Could you check a few things on this model? Use its own coordinates, in mm. A direction names the side the tool comes from. Give positions to 0.01 mm unless a question says otherwise; leave off trailing zeros. Loops run counter-clockwise (first coordinate to the right, second up) from the corner with the lowest first, then second, coordinate; pieces in that order, holes last. Notation, with made-up numbers: (82.5, 62) - (140.5, 62) arc R14 ccw to (140.5, 68) - close; hole circle Ø6 at (41.5, 86). An arc over 180 degrees is marked (long way). Use CSV: the item, a comma, the result in double quotes.
from build123d import *

# Parameters (mm, degrees)
EXTRUDE_1_DEPTH     = 20
SKETCH_2_R          = 1.5
CUT_EXTRUDE_1_DEPTH = 4
SKETCH_3_R          = 4
CUT_EXTRUDE_2_DEPTH = 4
SKETCH_4_R          = 1.5
CUT_EXTRUDE_3_DEPTH = 20
SKETCH_5_W          = 3
SKETCH_5_H          = 20
CUT_EXTRUDE_4_DEPTH = 8
SKETCH_6_W          = 20
SKETCH_6_H          = 27
CUT_EXTRUDE_5_DEPTH = 1
SKETCH_7_W          = 18
SKETCH_7_H          = 20
CUT_EXTRUDE_6_DEPTH = 1


with BuildPart() as part:
    # 草图1 → 凸台-拉伸1 (new body)
    with BuildSketch(Plane.XY):
        Polygon((0, 0), (0, 38), (3, 38), (3, 3), (20, 3), (20, 0), align=None)
    extrude(amount=EXTRUDE_1_DEPTH)

    # 草图2 → 切除-拉伸1 (cut, through all)
    with BuildSketch(Plane(origin=(0, 3, 0), x_dir=(1, 0, 0), z_dir=(0, 1, 0))):
        with Locations((16, -16)):
            Circle(SKETCH_2_R)
        with Locations((16, -4)):
            Circle(SKETCH_2_R)
    extrude(amount=-CUT_EXTRUDE_1_DEPTH, mode=Mode.SUBTRACT)

    # 草图3 → 切除-拉伸2 (cut, through all)
    with BuildSketch(Plane(origin=(3, 0, 0), x_dir=(0, 0, -1), z_dir=(1, 0, 0))):
        with Locations((-10, 18)):
            Circle(SKETCH_3_R)
    extrude(amount=-CUT_EXTRUDE_2_DEPTH, mode=Mode.SUBTRACT)

    # 草图4 → 切除-拉伸3 (cut)
    with BuildSketch(Plane(origin=(0, 3, 0), x_dir=(1, 0, 0), z_dir=(0, 1, 0))):
        with Locations((8, -16)):
            Circle(SKETCH_4_R)
        with Locations((8, -4)):
            Circle(SKETCH_4_R)
    extrude(amount=-CUT_EXTRUDE_3_DEPTH, mode=Mode.SUBTRACT)

    # 草图5 → 切除-拉伸4 (cut)
    with BuildSketch(Plane(origin=(0, 38, 0), x_dir=(1, 0, 0), z_dir=(0, 1, 0))):
        with Locations((1.5, -10)):
            Rectangle(SKETCH_5_W, SKETCH_5_H)
    extrude(amount=-CUT_EXTRUDE_4_DEPTH, mode=Mode.SUBTRACT)

    # 草图6 → 切除-拉伸5 (cut)
    with BuildSketch(Plane(origin=(3, 0, 0), x_dir=(0, 0, -1), z_dir=(1, 0, 0))):
        with Locations((-10, 16.5)):
            Rectangle(SKETCH_6_W, SKETCH_6_H)
    extrude(amount=-CUT_EXTRUDE_5_DEPTH, mode=Mode.SUBTRACT)

    # 草图7 → 切除-拉伸6 (cut)
    with BuildSketch(Plane(origin=(0, 3, 0), x_dir=(1, 0, 0), z_dir=(0, 1, 0))):
        with Locations((11, -10)):
            Rectangle(SKETCH_7_W, SKETCH_7_H)
    extrude(amount=-CUT_EXTRUDE_6_DEPTH, mode=Mode.SUBTRACT)


solid = part.part
1) Suppose I cut it at D-D (z = 10). Please give me the cut outline in (x, y).
Answer below:
outline,"(0, 0) - (20, 0) - (20, 2) - (2, 2) - (2, 14) - (0, 14) - close; (0, 22) - (2, 22) - (2, 30) - (0, 30) - close"
2) Suppose I cut it at C-C (x = 16). Please give me the cut outline in (y, z).
Answer below:
outline,"(0, 0) - (2, 0) - (2, 2.5) - (0, 2.5) - close; (0, 5.5) - (2, 5.5) - (2, 14.5) - (0, 14.5) - close; (0, 17.5) - (2, 17.5) - (2, 20) - (0, 20) - close"
3) Suppose I cut it at A-A (z = 16). Please give me the cut outline in (x, y).
Answer below:
outline,"(0, 0) - (6.5, 0) - (6.5, 2) - (2, 2) - (2, 30) - (0, 30) - close; (9.5, 0) - (14.5, 0) - (14.5, 2) - (9.5, 2) - close; (17.5, 0) - (20, 0) - (20, 2) - (17.5, 2) - close"
4) We'd pull the mould along Z, two halves only. Please class faces 1 (the cylindrical face through (14.5, 1.01, 15.93)), 2 (the flat face through (2, 13, 10)), 3 (the flat face through (1, 10, 0)): +Z half, -Z half, draft (parallel to the pull), parting line (faces both ways), or undercut.
Answer below:
face 1,"undercut"
face 2,"draft"
face 3,"-Z half"
5) Which directions (+Z, -Z, +X, -X, +Y, -Y) give clear straight access to the entire face, cutting with the end or side of a thin tool? Please do faces 4 (the flat face through (11, 2, 10)), 5 (the cylindrical face through (14.5, 1.01, 3.93)).
Answer below:
face 4,"+Z, -Z, +X, +Y"
face 5,"+Y, -Y"
6) I'm going to push flat-ended pins straight in: P1, Ø1.5, axis at y = 27, z = 16, coming from the -X side; P2, Ø2.5, axis at x = 8, z = 16, coming from the +Y side; P3, Ø5, axis at y = 13.5, z = 2.5, coming from the +X side; P4, Ø5.5, axis at x = 6.5, z = 8.5, coming from the +Y side. Where does each tip first touch, or does it pass through?
Answer below:
P1,"stops at x = 0"
P2,"passes through"
P3,"stops at x = 2"
P4,"stops at y = 2"
7) Suppose I cut it at B-B (y = 18). Please give me the cut outline in (x, z), plus the area to 3 significant figures.
Answer below:
outline,"(0, 0) - (2, 0) - (2, 6) - (0, 6) - close; (0, 14) - (2, 14) - (2, 20) - (0, 20) - close"
area,"24.0 mm2"
8) I need wall thicknesses on line 1 along Z through (x, y) = (8, 1.2); line 2 along X through (y, z) = (1.3, 16); line 3 along Y through (x, z) = (1.4, 10). Which ranges of each line are inside material? Lowest first, please.
Answer below:
line 1,"z = 0 to 2.5, 5.5 to 14.5, 17.5 to 20"
line 2,"x = 0 to 6.5, 9.5 to 14.5, 17.5 to 20"
line 3,"y = 0 to 14, 22 to 30"
